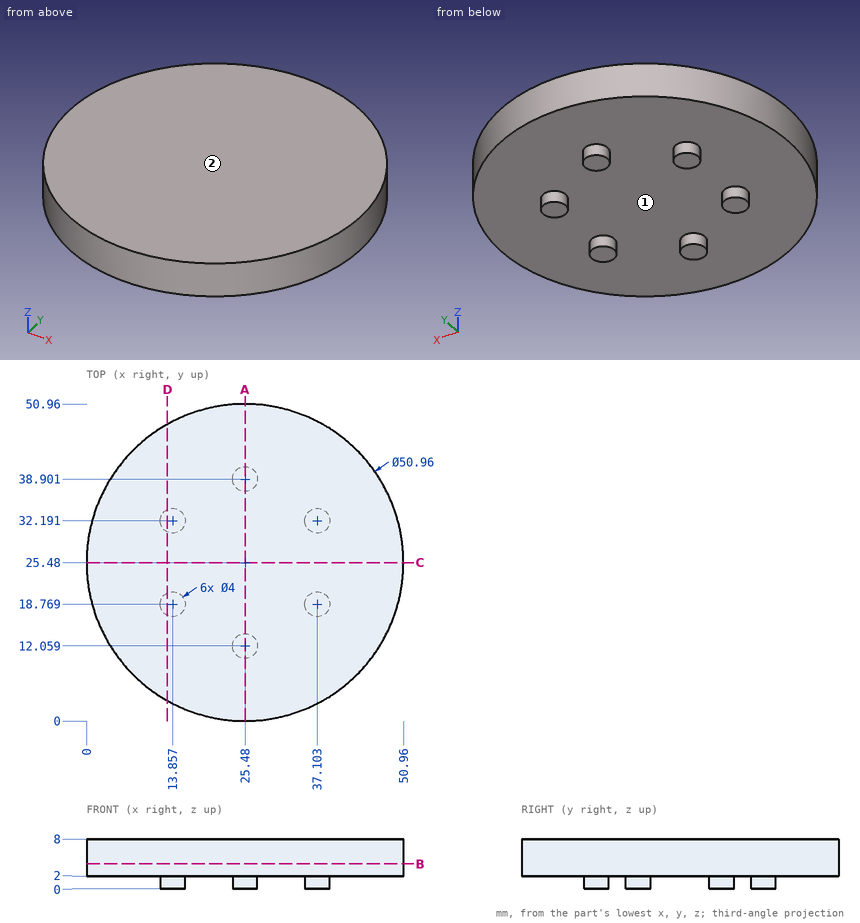
Check sheet for the drawn part. Datum: minimum x, y, z corner. Units: mm. A direction names the side the tool comes from. Round coordinates to 2 decimals unless told otherwise and drop trailing zeros. Loops run counter-clockwise (first coordinate to the right, second up) from the corner with the lowest first, then second, coordinate; pieces in that order, holes last. Notation, with made-up numbers: (-21, 68.5) - (20, 68.5) arc R9 ccw to (20, 81.5) - close; hole circle Ø11 at (22.25, 19.5). An arc over 180 degrees is marked (long way). Answer as a JSON object with one key per item and string values. Group by question number.
Q1. Sectioned sample at B-B, the plane z = 4. Enter the section's corners in (x, y), plus the area to 3 significant figures.
Q2. Sectioned sample at A-A, the plane x = 25.48. Enter the section's corners in (y, z).
Q3. Sectioned sample at C-C, the plane y = 25.48. Enter the section's corners in (x, z).
Q4. Gauge pin test, flat end, axial feed: P1, Ø3, axis at x = 36, z = 3, coming from the +Y side. Record the tip position at first contact, or that the pin passes through.
Q5. Sectioned sample at D-D, the plane x = 13. Enter the section's corners in (y, z) (1 decimal), plus the area to 3 significant figures.
Q6. Set-up check for the marked faces 1 and 2: record each of +Z, -Z, +X, -X, +Y, -Y from which the full face is reachable in a straight line by a thin tool's end or side.
Q7. Scan lines: line 1 along X through (y, z) = (32, 0.5) (1 decimal); line 2 along Z through (x, y) = (29, 34.5); line 3 along Y through (x, z) = (12.5, 1.5). Record each from-to range of solid material in increasing order. Write a range as [from, to].
Solution:
{
 "1": {"outline": "circle Ø50.96 at (25.48, 25.48)", "area": "2,040 mm²"},
 "2": {"outline": "(0, 2) - (10.06, 2) - (10.06, 0) - (14.06, 0) - (14.06, 2) - (36.9, 2) - (36.9, 0) - (40.9, 0) - (40.9, 2) - (50.96, 2) - (50.96, 8) - (0, 8) - close"},
 "3": {"outline": "(0, 2) - (50.96, 2) - (50.96, 8) - (0, 8) - close"},
 "4": {"P1": "stops at y = 49.31"},
 "5": {"outline": "(3.3, 2) - (17, 2) - (17, 0) - (20.6, 0) - (20.6, 2) - (30.4, 2) - (30.4, 0) - (34, 0) - (34, 2) - (47.7, 2) - (47.7, 8) - (3.3, 8) - close", "area": "281 mm²"},
 "6": {"face 1": "-Z", "face 2": "+Z, +X, -X, +Y, -Y"},
 "7": {"line 1": "x = [11.9, 15.8], [35.1, 39.1]", "line 2": "z = [2, 8]", "line 3": "y = [17.3, 20.24], [30.72, 33.66]"}
}
